Part print with two shaded views. Sizes in mm from the minimum x, y, z corner. Round coordinates to 2 decimals unless told otherwise and drop trailing zeros. Order: outer loops, then holes, each group sorted by start corner. A loop starts at its lowest first (then second) coordinate and runs counter-clockwise, first axis right, second up. Notation, with made-up numbers: M 38.25,72.25 L 56.25,72.25 A25 ccw 56.25,93.25 Z; hole C -22.75,54 d2. An arc over 180 degrees is marked long. Answer as a JSON object with one key per item and string values.
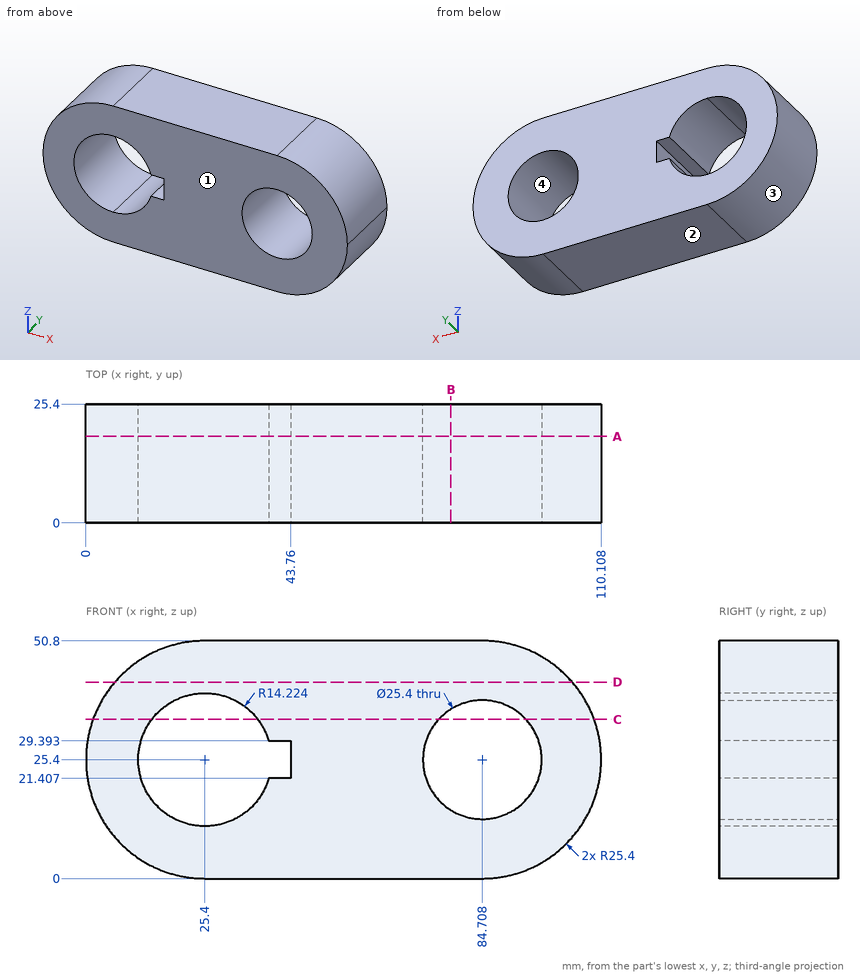
Item 1: Saw through at B-B on x = 78. List the corners of the cut face in (y, z) (1 decimal).
Worked answers:
{"outline": "M 0,0 L 25.4,0 L 25.4,14.6 L 0,14.6 Z; M 0,36.2 L 25.4,36.2 L 25.4,50.8 L 0,50.8 Z"}
Item 2: Drop flat-ended pins along their axis: pin 1 Ø6 at (y, z) = (4.5, 34.5) entering from -X; pin 2 Ø6 at (y, z) = (15.5, 6) entering from -X (1 decimal); pin 3 Ø2 at (y, z) = (13.5, 29.5) entering from +X; pin 4 Ø20.5 at (x, z) = (84.71, 25.4) entering from -Y. Give the stop position or say it passes through.
Worked answers:
{"pin 1": "stops at x = 0.74", "pin 2": "stops at x = 6", "pin 3": "stops at x = 109.92", "pin 4": "passes through"}
Item 3: Two-plate mould, pull along Z, no slides. Class the marked faces 1, 2, 3 and 4: released by +Z, released by -Z, zero draft, split by the parting line, or undercut.
Worked answers:
{"face 1": "zero draft", "face 2": "released by -Z", "face 3": "split by the parting line", "face 4": "undercut"}
Item 4: Saw through at D-D on z = 42. List the corners of the cut face in (x, y) (1 decimal).
Worked answers:
{"outline": "M 6.2,0 L 103.9,0 L 103.9,25.4 L 6.2,25.4 Z"}
Item 5: Saw through at C-C on z = 34. List the corners of the cut face in (x, y), and give its area (3 significant figures).
Worked answers:
{"outline": "M 1.5,0 L 14.07,0 L 14.07,25.4 L 1.5,25.4 Z; M 36.73,0 L 75.36,0 L 75.36,25.4 L 36.73,25.4 Z; M 94.05,0 L 108.61,0 L 108.61,25.4 L 94.05,25.4 Z", "area": "1,670 mm2"}
Item 6: Saw through at A-A on y = 18.5. List the corners of the cut face in (x, z).
Worked answers:
{"outline": "M 25.4,0 L 84.71,0 A25.4 ccw 84.71,50.8 L 25.4,50.8 A25.4 ccw Z; hole M 39.05,21.41 L 43.76,21.41 L 43.76,29.39 L 39.05,29.39 A14.22 ccw long Z; hole C 84.71,25.4 d25.4"}
Item 7: Wall check: line 1 along X through (y, z) = (8, 25.5); line 2 along X through (y, z) = (6.5, 19.5) (1 decimal); line 3 along Z through (x, y) = (31.5, 5). Give the ranges that are in metal, low to high. Write a range as [from, to].
Worked answers:
{"line 1": "x = [0, 11.18], [43.76, 72.01], [97.41, 110.11]", "line 2": "x = [0.7, 12.5], [38.3, 73.5], [96, 109.4]", "line 3": "z = [0, 12.55], [38.25, 50.8]"}
